The model under review builds one solid part; all positions refer to its coordinate system, in mm. Face numbers are marked on the shaded views. A direction names the side the tool comes from. Coordinates: 2 decimals unless noted, no trailing zeros. Write each loop counter-clockwise with the first axis right and the second up, starting at its lowest first coordinate (ties: lowest second). Pieces come first, ordered by that corner, then holes. Notation, with made-up numbers: (-23.75, -19.75) - (4.25, -19.75) arc R27 cw to (4.25, 14.25) - close; hole circle Ø2 at (-23, 36.5). An arc over 180 degrees is marked (long way). Return JSON: item names as keys, results as strings. Group by question number.
(1) We need section D-D on y = 18.5. State the section outline as (x, z) points, then the cut area to 3 significant figures.
(2) To check wall thickness, follow L1, parallel to Y at x = 15, z = 4.5; L2, parallel to Y at x = -6, z = -2; L3, parallel to X at y = 13, z = 3.5. State the ranges of each line that lie inside material, in increasing order. Write a range as from..to.
(3) We need section B-B on y = 33.5. Give the number of separate pieces and of enclosed holes in the cut face, then the cut area to 3 significant figures.
(4) For pin 1 Ø1.5 at (x, z) = (14, 8.5) entering from +Y; pin 2 Ø8 at (x, y) = (-15.5, 13.5) entering from -Z; pin 3 Ø6 at (x, z) = (-5, -7) entering from +Y; pin 4 Ø8 at (y, z) = (29.5, -10) entering from -X, all flat-tipped, find the tip position at first contact; note any pin that passes through.
(5) Draft analysis for pull direction Z (two halves, no side actions). For the marked faces 3, 4 and 5, state which applies: released by +Z, released by -Z, zero draft, split by the parting line, or undercut.
(6) We need section C-C on z = 2. State the section outline as (x, y) points, then the cut area to 4 significant figures.
(7) We need section A-A on x = -16. State the section outline as (y, z) points.
(8) Tool access review of the marked faces 1 and 2: name each direction out of +Z, -Z, +X, -X, +Y, -Y from which nothing blocks a thin tool from reaching the whole face with its end or side.
```python
from build123d import *

# Parameters (mm, degrees)
SKETCH_1_W                  = 21.875
SKETCH_1_H                  = 2.5
SKETCH_2_R                  = 10.9
EXTRUDE_1_DEPTH             = 25.75
HOLE_WIZARD_M18_1_D         = 19.2
HOLE_WIZARD_M18_1_DEPTH     = 1.6
SKETCH_5_W                  = 8.1
SKETCH_5_H                  = 1.6
SKETCH_6_W                  = 0.4
SKETCH_6_H                  = 10
SKETCH_7_W                  = 0.4
SKETCH_7_H                  = 10
SKETCH_8_W                  = 0.4
SKETCH_8_H                  = 10
SKETCH_9_W                  = 0.4
SKETCH_9_H                  = 10
SKETCH_10_W                 = 0.4
SKETCH_10_H                 = 10
SKETCH_11_W                 = 0.4
SKETCH_11_H                 = 10
SKETCH_12_W                 = 0.4
SKETCH_12_H                 = 10
SKETCH_13_W                 = 0.4
SKETCH_13_H                 = 10
SKETCH_14_W                 = 0.4
SKETCH_14_H                 = 10
SKETCH_15_W                 = 0.4
SKETCH_15_H                 = 10
SKETCH_16_W                 = 0.4
SKETCH_16_H                 = 10
SKETCH_17_W                 = 0.4
SKETCH_17_H                 = 10
HOLE_WIZARD_5_4_5_4_1_D     = 5.4
HOLE_WIZARD_9_5_9_5_1_D     = 9.5
HOLE_WIZARD_9_5_9_5_1_DEPTH = 0.5


with BuildPart() as part:
    # 草图1 → 旋转1 (revolve)
    with BuildSketch(Plane.XY, mode=Mode.PRIVATE) as revolve_1_sk:
        with Locations((10.9375, 1.25)):
            Rectangle(SKETCH_1_W, SKETCH_1_H)
    revolve(revolve_1_sk.sketch.rotate(Axis((0, 2.5, 0), (0, -1, 0)), 270), axis=Axis((0, 2.5, 0), (0, -1, 0)))

    # 草图2 → 凸台-拉伸1 (add)
    with BuildSketch(Plane(origin=(0, 2.5, 0), x_dir=(-1, 0, 0), z_dir=(0, 1, 0))):
        with Locations(Location((0, 0, 0), (0, 0, 90))):
            Circle(SKETCH_2_R)
    extrude(amount=EXTRUDE_1_DEPTH)

    # M18 间隙孔1
    with Locations(Plane(origin=(0, 0, 0), x_dir=(-1, 0, 0), z_dir=(0, -1, 0))):
        with Locations((0, 0)):
            Hole(HOLE_WIZARD_M18_1_D / 2, depth=HOLE_WIZARD_M18_1_DEPTH)

    # 草图5 → 旋转2 (revolve)
    with BuildSketch(Plane.XY, mode=Mode.PRIVATE) as revolve_2_sk:
        with Locations((4.05, 0.8)):
            Rectangle(SKETCH_5_W, SKETCH_5_H)
    revolve(revolve_2_sk.sketch.rotate(Axis((0, 1.6, 0), (0, -1, 0)), 270), axis=Axis((0, 1.6, 0), (0, -1, 0)))

    # 草图6 → 旋转3 (revolve)
    with BuildSketch(Plane.XY.offset(9.847808943), mode=Mode.PRIVATE) as revolve_3_sk:
        with Locations((1.938004324, 33.25)):
            Rectangle(SKETCH_6_W, SKETCH_6_H)
    revolve(revolve_3_sk.sketch.rotate(Axis((1.738004324, 38.25, 9.847808943), (0, -1, 0)), 270), axis=Axis((1.738004324, 38.25, 9.847808943), (0, -1, 0)))

    # 草图7 → 旋转4 (revolve)
    with BuildSketch(Plane.XY.offset(9.854071628), mode=Mode.PRIVATE) as revolve_4_sk:
        with Locations((-1.502137581, 33.25)):
            Rectangle(SKETCH_7_W, SKETCH_7_H)
    revolve(revolve_4_sk.sketch.rotate(Axis((-1.702137581, 38.25, 9.854071628), (0, -1, 0)), 270), axis=Axis((-1.702137581, 38.25, 9.854071628), (0, -1, 0)))

    # 草图8 → 旋转5 (revolve)
    with BuildSketch(Plane.XY.offset(9.961946981), mode=Mode.PRIVATE) as revolve_5_sk:
        with Locations((-0.671557427, 33.25)):
            Rectangle(SKETCH_8_W, SKETCH_8_H)
    revolve(revolve_5_sk.sketch.rotate(Axis((-0.871557427, 38.25, 9.961946981), (0, -1, 0)), 270), axis=Axis((-0.871557427, 38.25, 9.961946981), (0, -1, 0)))

    # 草图9 → 旋转6 (revolve)
    with BuildSketch(Plane.XY.offset(9.961946981), mode=Mode.PRIVATE) as revolve_6_sk:
        with Locations((1.071557427, 33.25)):
            Rectangle(SKETCH_9_W, SKETCH_9_H)
    revolve(revolve_6_sk.sketch.rotate(Axis((0.871557427, 38.25, 9.961946981), (0, -1, 0)), 270), axis=Axis((0.871557427, 38.25, 9.961946981), (0, -1, 0)))

    # 草图10 → 旋转7 (revolve)
    with BuildSketch(Plane.XY.offset(10), mode=Mode.PRIVATE) as revolve_7_sk:
        with Locations((0.2, 33.25)):
            Rectangle(SKETCH_10_W, SKETCH_10_H)
    revolve(revolve_7_sk.sketch.rotate(Axis((0, 38.25, 10), (0, -1, 0)), 270), axis=Axis((0, 38.25, 10), (0, -1, 0)))

    # 草图11 → 旋转8 (revolve)
    with BuildSketch(Plane.XY.offset(-9.670983902), mode=Mode.PRIVATE) as revolve_8_sk:
        with Locations((2.744026408, 33.25)):
            Rectangle(SKETCH_11_W, SKETCH_11_H)
    revolve(revolve_8_sk.sketch.rotate(Axis((2.544026408, 38.25, -9.670983902), (0, -1, 0)), 270), axis=Axis((2.544026408, 38.25, -9.670983902), (0, -1, 0)))

    # 草图12 → 旋转9 (revolve)
    with BuildSketch(Plane.XY.offset(-9.847808943), mode=Mode.PRIVATE) as revolve_9_sk:
        with Locations((1.938004324, 33.25)):
            Rectangle(SKETCH_12_W, SKETCH_12_H)
    revolve(revolve_9_sk.sketch.rotate(Axis((1.738004324, 38.25, -9.847808943), (0, -1, 0)), 270), axis=Axis((1.738004324, 38.25, -9.847808943), (0, -1, 0)))

    # 草图13 → 旋转10 (revolve)
    with BuildSketch(Plane.XY.offset(-9.854071628), mode=Mode.PRIVATE) as revolve_10_sk:
        with Locations((-1.502137581, 33.25)):
            Rectangle(SKETCH_13_W, SKETCH_13_H)
    revolve(revolve_10_sk.sketch.rotate(Axis((-1.702137581, 38.25, -9.854071628), (0, -1, 0)), 270), axis=Axis((-1.702137581, 38.25, -9.854071628), (0, -1, 0)))

    # 草图14 → 旋转11 (revolve)
    with BuildSketch(Plane.XY.offset(-9.961946981), mode=Mode.PRIVATE) as revolve_11_sk:
        with Locations((-0.671557427, 33.25)):
            Rectangle(SKETCH_14_W, SKETCH_14_H)
    revolve(revolve_11_sk.sketch.rotate(Axis((-0.871557427, 38.25, -9.961946981), (0, -1, 0)), 270), axis=Axis((-0.871557427, 38.25, -9.961946981), (0, -1, 0)))

    # 草图15 → 旋转12 (revolve)
    with BuildSketch(Plane.XY.offset(-9.961946981), mode=Mode.PRIVATE) as revolve_12_sk:
        with Locations((1.071557427, 33.25)):
            Rectangle(SKETCH_15_W, SKETCH_15_H)
    revolve(revolve_12_sk.sketch.rotate(Axis((0.871557427, 38.25, -9.961946981), (0, -1, 0)), 270), axis=Axis((0.871557427, 38.25, -9.961946981), (0, -1, 0)))

    # 草图16 → 旋转13 (revolve)
    with BuildSketch(Plane.XY.offset(-10), mode=Mode.PRIVATE) as revolve_13_sk:
        with Locations((0.2, 33.25)):
            Rectangle(SKETCH_16_W, SKETCH_16_H)
    revolve(revolve_13_sk.sketch.rotate(Axis((0, 38.25, -10), (0, -1, 0)), 270), axis=Axis((0, 38.25, -10), (0, -1, 0)))

    # 草图17 → 旋转14 (revolve)
    with BuildSketch(Plane.XY.offset(9.670983902), mode=Mode.PRIVATE) as revolve_14_sk:
        with Locations((2.744026408, 33.25)):
            Rectangle(SKETCH_17_W, SKETCH_17_H)
    revolve(revolve_14_sk.sketch.rotate(Axis((2.544026408, 38.25, 9.670983902), (0, -1, 0)), 270), axis=Axis((2.544026408, 38.25, 9.670983902), (0, -1, 0)))

    # Ø5.4 (5.4) 直径孔1 (through all)
    with Locations(Plane(origin=(0, 2.5, 0), x_dir=(1, 0, 0), z_dir=(0, 1, 0))):
        with Locations((0, -17.425), (-15.090492661, 8.7125), (15.090492661, 8.7125)):
            Hole(HOLE_WIZARD_5_4_5_4_1_D / 2)

    # Ø9.5 (9.5) 直径孔1
    with Locations(Plane(origin=(0, 0, 0), x_dir=(-1, 0, 0), z_dir=(0, -1, 0))):
        with Locations((0, 0)):
            Hole(HOLE_WIZARD_9_5_9_5_1_D / 2, depth=HOLE_WIZARD_9_5_9_5_1_DEPTH)


solid = part.part
```
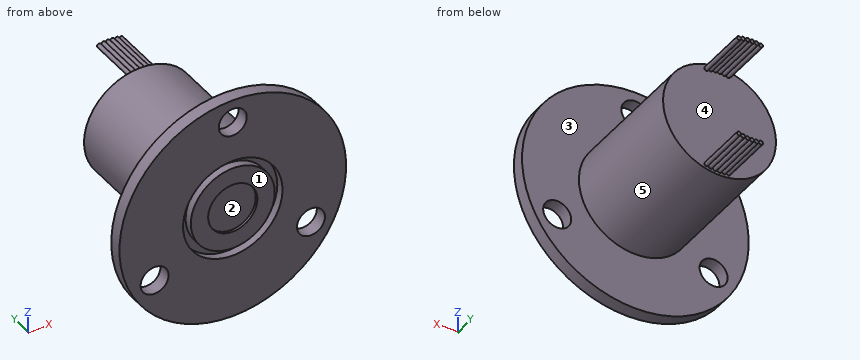
Ans:
{
 "1": {"outline": "circle Ø21.8 at (0, 0)", "area": "373 mm²"},
 "2": {"L1": "0..2.5", "L2": "0..28.25", "L3": "-10.32..10.32"},
 "3": {"separate pieces": "12", "enclosed holes": "0", "area": "6.03 mm²"},
 "4": {"pin 1": "y = 2.5", "pin 2": "through", "pin 3": "y = 28.25", "pin 4": "x = -8.96"},
 "5": {"face 3": "zero draft", "face 4": "undercut", "face 5": "split by the parting line"},
 "6": {"outline": "(-21.78, 0) - (-9.39, 0) - (-9.39, 1.6) - (-7.85, 1.6) - (-7.85, 0) - (-4.31, 0) - (-4.31, 0.5) - (4.31, 0.5) - (4.31, 0) - (7.85, 0) - (7.85, 1.6) - (9.39, 1.6) - (9.39, 0) - (21.78, 0) - (21.78, 2.5) - (10.71, 2.5) - (10.71, 28.25) - (-10.71, 28.25) - (-10.71, 2.5) - (-21.78, 2.5) - close", "area": "651.5 mm²"},
 "7": {"outline": "(0, -14.92) - (2.5, -14.92) - (2.5, -11.25) - (0, -11.25) - close; (0, -6.17) - (2.5, -6.17) - (2.5, 14.92) - (0, 14.92) - close"},
 "8": {"face 1": "+Z, -Z, +X, -X, -Y", "face 2": "-Y"}
}
